Design review of the part built by this model. Coordinates are the model's own, in mm. Face numbers are marked on the shaded views. A direction names the side the tool comes from. Give positions to 0.01 mm unless a question says otherwise; leave off trailing zeros. Loops run counter-clockwise (first coordinate to the right, second up) from the corner with the lowest first, then second, coordinate; pieces in that order, holes last. Notation, with made-up numbers: (-17.5, 30.5) -> (16.5, 30.5) arc R8 ccw to (16.5, 45.5) -> close; hole circle Ø1 at (-3.5, 9). An arc over 180 degrees is marked (long way). Use CSV: the item, a comma, the result in double quotes. Start each with the question number.
Item 1: We need section B-B (z = -23.5). State the section outline as (x, y) points, plus the area to 3 significant figures.
Item 2: We need section D-D (z = -12.75). State the section outline as (x, y) points, plus the area to 3 significant figures.
Item 3: We need section A-A (y = 16). State the section outline as (x, z) points.
Item 4: We need section C-C (x = 52.5). State the section outline as (y, z) points, plus the area to 3 significant figures.
Item 5: Wall thickness on line 1 along X through (y, z) = (2.85, -12.75); line 2 along X through (y, z) = (18.5, -50); line 3 along Z through (x, y) = (52.5, 1.75): over which ranges is each line inside the solid? List them lowest first. Write a range as from..to.
Item 6: Clearance check with flat-ended pins moving along their axes: pin 1 (6 mm diameter, centred on x = 58.5, y = 9.5, fed in from +Z); pin 2 (12.5 mm diameter, centred on x = 44, z = -13, fed in from +Y); pin 3 (3 mm diameter, centred on y = 18, z = -51.5, fed in from -X). State where each tip first meets the part, or that it passes through.
Item 7: For the marked faces 1 and 2, list the 3-axis set-ups (+Z, -Z, +X, -X, +Y, -Y) from which the entire face can be reached by the end or side of a thin tool; tool diameter is ignored.
from build123d import *

# Parameters (mm, degrees)
SKETCH1_R                = 2.55
BOSS_EXTRUDE1_DEPTH      = 4
SKETCH2_R                = 2
SKETCH2_W                = 65
SKETCH2_H                = 4
BOSS_EXTRUDE2_DEPTH      = 13
BOSS_EXTRUDE3_DEPTH      = 4
SKETCH4_W                = 65
SKETCH4_H                = 4
BOSS_EXTRUDE4_DEPTH      = 20
FILLET1_R                = 4
SKETCH6_R                = 2.55
CUT_EXTRUDE1_DEPTH       = 20
SKETCH7_W                = 46
SKETCH7_H                = 4
CUT_EXTRUDE2_DEPTH       = 80
BOSS_EXTRUDE6_DEPTH      = 2.5
BOSS_EXTRUDE6_DEPTH_BACK = 2.5
CUT_EXTRUDE3_REACH       = 94.25
FILLET2_R                = 4
SKETCH8_R                = 6
SKETCH8_R_2              = 2.5
BOSS_EXTRUDE5_DEPTH      = 5
FILLET3_R                = 4
BOSS_EXTRUDE7_START      = 4
BOSS_EXTRUDE7_DEPTH      = 3.5
SKETCH13_R               = 4.5
CUT_EXTRUDE4_DEPTH       = 6
SKETCH14_W               = 13.282344927
SKETCH14_H               = 18
CUT_EXTRUDE5_DEPTH       = 6
FILLET5_R                = 4


with BuildPart() as part:
    # Sketch1 → Boss-Extrude1 (new body)
    with BuildSketch(Plane(origin=(0, 0, 0), x_dir=(1, 0, 0), z_dir=(0, 1, 0))):
        with BuildLine():
            Line((4, 0), (61, 0))
            ThreePointArc((61, 0), (63.828427125, 1.171572875), (65, 4))
            Line((65, 4), (65, 42))
            Line((65, 42), (0, 42))
            Line((0, 42), (0, 4))
            ThreePointArc((0, 4), (1.171572875, 1.171572875), (4, 0))
        make_face()
        with Locations(Location((12.5, 12.75, 0), (0, 0, 270))):
            Circle(SKETCH1_R, mode=Mode.SUBTRACT)
        with Locations(Location((52.5, 12.75, 0), (0, 0, 270))):
            Circle(SKETCH1_R, mode=Mode.SUBTRACT)
    extrude(amount=BOSS_EXTRUDE1_DEPTH)

    # Sketch2 → Boss-Extrude2 (add)
    with BuildSketch(Plane(origin=(0, 4, 0), x_dir=(1, 0, 0), z_dir=(0, 1, 0))):
        with Locations(Location((61, 4, 0), (0, 0, 90))):
            Circle(SKETCH2_R)
        with Locations(Location((4, 4, 0), (0, 0, 90))):
            Circle(SKETCH2_R)
        with Locations((32.5, 40)):
            Rectangle(SKETCH2_W, SKETCH2_H)
    extrude(amount=BOSS_EXTRUDE2_DEPTH)

    # Sketch3 → Boss-Extrude3 (add)
    with BuildSketch(Plane(origin=(0, 17, 0), x_dir=(1, 0, 0), z_dir=(0, 1, 0))):
        with BuildLine():
            Line((0, 42), (65, 42))
            Line((65, 42), (65, 4))
            ThreePointArc((65, 4), (63.828427125, 1.171572875), (61, 0))
            Line((61, 0), (4, 0))
            ThreePointArc((4, 0), (1.171572875, 1.171572875), (0, 4))
            Line((0, 4), (0, 42))
        make_face()
    extrude(amount=BOSS_EXTRUDE3_DEPTH)

    # Sketch4 → Boss-Extrude4 (add)
    with BuildSketch(Plane(origin=(0, 0, -42), x_dir=(-1, 0, 0), z_dir=(0, 0, -1))):
        with Locations((-32.5, 19)):
            Rectangle(SKETCH4_W, SKETCH4_H)
    extrude(amount=BOSS_EXTRUDE4_DEPTH)

    # Fillet1
    fillet1_edges = [part.edges().sort_by_distance(p)[0] for p in [
        (65, 19, -62),
        (0, 19, -62),
    ]]
    fillet(fillet1_edges, radius=FILLET1_R)

    # Sketch6 → Cut-Extrude1 (cut)
    with BuildSketch(Plane(origin=(0, 21, 0), x_dir=(1, 0, 0), z_dir=(0, 1, 0))):
        with Locations(Location((57.65, 50.10433299, 0), (0, 0, 270))):
            Circle(SKETCH6_R)
        with Locations(Location((45.5, 32.10433299, 0), (0, 0, 270))):
            Circle(SKETCH6_R)
    extrude(amount=-CUT_EXTRUDE1_DEPTH, mode=Mode.SUBTRACT)

    # Sketch7 → Cut-Extrude2 (cut)
    with BuildSketch(Plane.XY):
        Polygon((4, 17), (4, 21), (0, 21), (0, 4), (50, 4), (50, 17), align=None)
        with Locations((27, 19)):
            Rectangle(SKETCH7_W, SKETCH7_H)
    extrude(amount=-CUT_EXTRUDE2_DEPTH, mode=Mode.SUBTRACT)

    # Sketch10 → Boss-Extrude6 (add, two sides: drawn at the far end of the back side and taken through both)
    with BuildSketch(Plane(origin=(57.5, 0, 0), x_dir=(0, 0, -1), z_dir=(1, 0, 0)).offset(-BOSS_EXTRUDE6_DEPTH_BACK)):
        Polygon((33, 4), (38, 9), (38, 4), align=None)
    extrude(amount=BOSS_EXTRUDE6_DEPTH + BOSS_EXTRUDE6_DEPTH_BACK)

    # Cut-Extrude3: up to this face of the body (flat: up to its plane)
    cut_extrude3_end = Plane(part.part.faces().sort_by_distance((31.428078694, 4, -20.594205602))[0])
    # Sketch11 → Cut-Extrude3 (cut, up to the picked face)
    with BuildSketch(Plane(origin=(0, 21, 0), x_dir=(1, 0, 0), z_dir=(0, 1, 0)), mode=Mode.PRIVATE) as cut_extrude3_sk1:
        with BuildLine():
            Line((57.5, 0), (57.5, 42))
            ThreePointArc((57.5, 42), (56.914213562, 43.414213562), (55.5, 44))
            Line((55.5, 44), (50, 44))
            Line((50, 44), (50, 0))
            Line((50, 0), (57.5, 0))
        make_face()
    cut_extrude3_tool1 = split(extrude(cut_extrude3_sk1.sketch, amount=-CUT_EXTRUDE3_REACH, mode=Mode.PRIVATE), bisect_by=cut_extrude3_end, keep=Keep.BOTH, mode=Mode.PRIVATE)
    add(cut_extrude3_tool1.solids().sort_by(Axis((53.741385, 21, -21.943789), (0, -1, 0)))[0], mode=Mode.SUBTRACT)

    # Fillet2
    # the kernel refuses this fillet: 4 mm, written as the material it takes off along each edge
    with BuildSketch(Plane(origin=(57.5, 30.921567416, 0), x_dir=(1, 0, 0), z_dir=(0, -1, 0))) as fillet2_piece_1:
        with BuildLine():
            CenterArc((4, -3.968626967), FILLET2_R, 97.180755781, 82.819244219)
            Line((0, -3.968626967), (-0.08, -3.968626967))
            Line((-0.08, -3.968626967), (-0.08, 0))
            Line((-0.08, 0), (0, 0.08))
            ThreePointArc((0, 0.08), (1.75, 0.08), (3.49, 0.079372539))
            Line((3.49, 0.079372539), (3.5, 0))
        make_face()
    extrude(amount=23.843134833, mode=Mode.SUBTRACT)

    # Sketch8 → Boss-Extrude5 (add)
    with BuildSketch(Plane(origin=(0, 4, 0), x_dir=(1, 0, 0), z_dir=(0, 1, 0))):
        with Locations(Location((45.5, 32.10433299, 0), (0, 0, 270))):
            Circle(SKETCH8_R)
        with Locations(Location((45.5, 32.10433299, 0), (0, 0, 270))):
            Circle(SKETCH8_R_2, mode=Mode.SUBTRACT)
    extrude(amount=BOSS_EXTRUDE5_DEPTH)

    # Fillet3
    fillet3_edges = [part.edges().sort_by_distance(p)[0] for p in [
        (50, 19, -62),
    ]]
    fillet(fillet3_edges, radius=FILLET3_R)

    # Sketch12 → Boss-Extrude7 (add)
    with BuildSketch(Plane(origin=(57.5, 0, 0), x_dir=(0, 0, -1), z_dir=(1, 0, 0)).offset(BOSS_EXTRUDE7_START)):
        Polygon((42, 12), (47, 17), (42, 17), align=None)
    extrude(amount=BOSS_EXTRUDE7_DEPTH)

    # Sketch13 → Cut-Extrude4 (cut)
    with BuildSketch(Plane.XZ):
        with Locations(Location((45.5, -32.10433299, 0), (0, 0, 270))):
            Circle(SKETCH13_R)
    extrude(amount=-CUT_EXTRUDE4_DEPTH, mode=Mode.SUBTRACT)

    # Sketch14 → Cut-Extrude5 (cut)
    with BuildSketch(Plane(origin=(0, 21, 0), x_dir=(1, 0, 0), z_dir=(0, 1, 0))):
        with Locations((47.623272126, 53)):
            Rectangle(SKETCH14_W, SKETCH14_H)
    extrude(amount=-CUT_EXTRUDE5_DEPTH, mode=Mode.SUBTRACT)

    # Fillet5
    fillet5_edges = [part.edges().sort_by_distance(p)[0] for p in [
        (54.264444589, 19, -62),
        (54.264444589, 19, -44),
    ]]
    fillet(fillet5_edges, radius=FILLET5_R)


solid = part.part
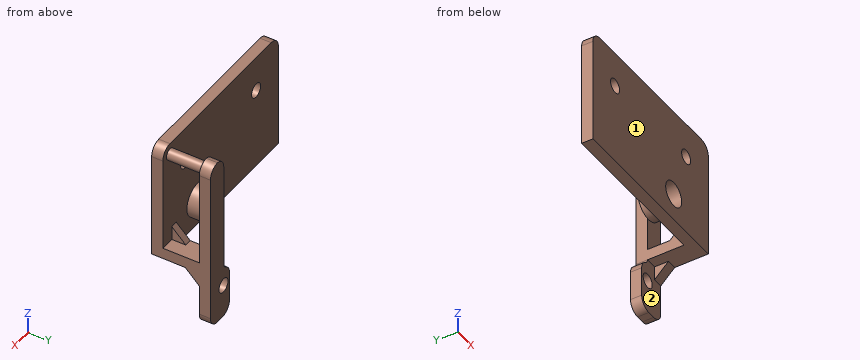
Results found:
1,outline,"(0, 0) -> (65, 0) -> (65, 4) -> (0, 4) -> close; (57.5, 17) -> (65, 17) -> (65, 21) -> (57.5, 21) -> close"
1,area,"290 mm²"
2,outline,"(0, 0) -> (9.95, 0) -> (9.95, 4) -> (0, 4) -> close; (15.05, 0) -> (49.95, 0) -> (49.95, 4) -> (15.05, 4) -> close; (55.05, 0) -> (65, 0) -> (65, 4) -> (55.05, 4) -> close; (57.5, 17) -> (65, 17) -> (65, 21) -> (57.5, 21) -> close"
2,area,"249 mm²"
3,outline,"(57.5, -42) -> (61.5, -42) -> (61.5, -46) -> (65, -46) -> (65, -38) -> (57.5, -38) -> close; circle Ø4 at (61, -4)"
4,outline,"(0, -42) -> (4, -42) -> (4, -15.3) -> (0, -15.3) -> close; (0, -10.2) -> (4, -10.2) -> (4, 0) -> (0, 0) -> close"
4,area,"148 mm²"
5,line 1,"0..9.95, 15.05..49.95, 55.05..65"
5,line 2,"54.26..55.1, 60.2..65"
5,line 3,"-42..-15.3, -10.2..0"
6,pin 1,"z = -2"
6,pin 2,"y = 4"
6,pin 3,"x = 54.26"
7,face 1,"+Z, -Z, +X, -X, -Y"
7,face 2,"-Z, -X, -Y"
